```python
from build123d import *

# Parameters (mm, degrees)
SKETCH_1_W             = 140
SKETCH_1_H             = 60
EXTRUDE_1_DEPTH        = 5
SKETCH_2_R             = 1.2
CUT_EXTRUDE_1096_DEPTH = 153.397506541
SKETCH_4_R             = 1.4
CUT_EXTRUDE_3_DEPTH    = 5
PATTERN_LINEAR_1_COUNT = 3
PATTERN_LINEAR_1_PITCH = 40
SKETCH_6_R             = 2
CUT_EXTRUDE_4_DEPTH    = 1


with BuildPart() as part:
    # Sketch 1 → Extrude 1 (new body)
    with BuildSketch(Plane(origin=(0, 0, 0), x_dir=(1, 0, 0), z_dir=(0, 1, 0))):
        with Locations((70, -30)):
            Rectangle(SKETCH_1_W, SKETCH_1_H)
    extrude(amount=EXTRUDE_1_DEPTH)

    # Sketch 2 → Cut-Extrude 1096 (cut, through all)
    with BuildSketch(Plane(origin=(0, 5, 0), x_dir=(1, 0, 0), z_dir=(0, 1, 0))):
        with Locations(Location((102, -15, 0), (0, 0, 270))):
            Circle(SKETCH_2_R)
        with Locations(Location((118, -15, 0), (0, 0, 270))):
            Circle(SKETCH_2_R)
        with Locations(Location((102, -45, 0), (0, 0, 90))):
            Circle(SKETCH_2_R)
        with Locations(Location((118, -45, 0), (0, 0, 90))):
            Circle(SKETCH_2_R)
        with BuildLine():
            Line((100, -26.05), (100, -36.95))
            Line((100, -36.95), (104.2, -36.95))
            Line((104.2, -36.95), (104.2, -29.381860214))
            ThreePointArc((104.2, -29.381860214), (110, -31.5), (115.8, -29.381860214))
            Line((115.8, -29.381860214), (115.8, -36.95))
            Line((115.8, -36.95), (120, -36.95))
            Line((120, -36.95), (120, -26.05))
            Line((120, -26.05), (118.270278109, -26.05))
            ThreePointArc((118.270278109, -26.05), (110, -13.5), (101.729721891, -26.05))
            Line((101.729721891, -26.05), (100, -26.05))
        make_face()
    cut_extrude_1096 = extrude(amount=-CUT_EXTRUDE_1096_DEPTH, mode=Mode.SUBTRACT)

    # Sketch 4 → Cut-Extrude 3 (cut)
    with BuildSketch(Plane.ZY):
        with Locations((30, 2.5)):
            Circle(SKETCH_4_R)
        with Locations((8, 2.5)):
            Circle(SKETCH_4_R)
        with Locations((52, 2.5)):
            Circle(SKETCH_4_R)
    cut_extrude_3 = extrude(amount=-CUT_EXTRUDE_3_DEPTH, mode=Mode.SUBTRACT)

    # Mirror 1: Cut-Extrude 3 across plane
    add(cut_extrude_3.mirror(Plane(origin=(70, 0, 0), x_dir=(0, 0, 1), z_dir=(1, 0, 0))), mode=Mode.SUBTRACT)

    # Pattern Linear 1: Cut-Extrude 1096 ×3
    with Locations(*[(-i * PATTERN_LINEAR_1_PITCH, 0, 0) for i in range(1, PATTERN_LINEAR_1_COUNT)]):
        add(cut_extrude_1096, mode=Mode.SUBTRACT)

    # Sketch 6 → Cut-Extrude 4 (cut)
    with BuildSketch(Plane.XZ):
        with Locations(Location((22, 45, 0), (0, 0, 270))):
            Circle(SKETCH_6_R)
        with Locations(Location((38, 45, 0), (0, 0, 270))):
            Circle(SKETCH_6_R)
        with Locations(Location((62, 45, 0), (0, 0, 270))):
            Circle(SKETCH_6_R)
        with Locations(Location((78, 45, 0), (0, 0, 270))):
            Circle(SKETCH_6_R)
        with Locations(Location((102, 45, 0), (0, 0, 270))):
            Circle(SKETCH_6_R)
        with Locations(Location((118, 45, 0), (0, 0, 270))):
            Circle(SKETCH_6_R)
        with Locations((22, 15)):
            Circle(SKETCH_6_R)
        with Locations((38, 15)):
            Circle(SKETCH_6_R)
        with Locations((62, 15)):
            Circle(SKETCH_6_R)
        with Locations((78, 15)):
            Circle(SKETCH_6_R)
        with Locations((102, 15)):
            Circle(SKETCH_6_R)
        with Locations((118, 15)):
            Circle(SKETCH_6_R)
    extrude(amount=-CUT_EXTRUDE_4_DEPTH, mode=Mode.SUBTRACT)


solid = part.part
```
Could you check a few things on this model? Use its own coordinates, in mm. A direction names the side the tool comes from. Round coordinates to 2 decimals unless told otherwise and drop trailing zeros. Loops run counter-clockwise (first coordinate to the right, second up) from the corner with the lowest first, then second, coordinate; pieces in that order, holes last.
Q1. I want a section at B-B (y = 2.5). Give the number of separate pieces and of enclosed holes in the cut face, and give its area (3 significant figures).
Q2. On a 3-axis mill with a long thin cutter (end or side, diameter ignored), from which of +Z, -Z, +X, -X, +Y, -Y can I reach the whole of each face in a straight line? I mean faces 1 (the flat face through (23, 1, 14)), 2 (the flat face through (104.2, 3, 33)), 3 (the cylindrical face through (137.54, 1.96, 53.29)). Say none if no direction works.
Q3. Please list where these lines run through material, in increasing order: L1, parallel to Z at x = 30, y = 1.8; L2, parallel to Y at x = 137, z = 52; L3, parallel to Z at x = 118, y = 3.2.
Q4. Thinking about a two-plate mould opening in X: for faces 4 (the flat face through (69, 5, 36)), 5 (the flat face through (135, 3, 30)), 6 (the cylindrical face through (60.99, 3.03, 44.35)), which applies, pulls with the +X half, pulls with the -X half, needs draft (parallel to the pull), parting line crosses it, or undercut?
Q5. For P1, Ø3, axis at x = 22, z = 15, coming from the -Y side; P2, Ø2, axis at x = 102, z = 45, coming from the -Y side, each with a flat end and sliding along its axis, tell me the tip position at first contact or that it passes through.
Q6. I want a section at A-A (z = 8). Write out the boundary of the cut face in (x, y), and give its area (3 significant figures).
Answer below:
1. separate pieces: 1
1. enclosed holes: 15
1. area: 7,250 mm2
2. face 1: -Y
2. face 2: +Y, -Y
2. face 3: +X
3. L1: z = 0 to 13.5, 31.5 to 60
3. L2: y = 0 to 1.1, 3.9 to 5
3. L3: z = 0 to 13.8, 16.2 to 18.38, 36.95 to 43.8, 46.2 to 60
4. face 4: needs draft
4. face 5: pulls with the +X half
4. face 6: undercut
5. P1: stops at y = 1
5. P2: passes through
6. outline: (0, 0) - (140, 0) - (140, 1.1) - (135, 1.1) - (135, 3.9) - (140, 3.9) - (140, 5) - (0, 5) - (0, 3.9) - (5, 3.9) - (5, 1.1) - (0, 1.1) - close
6. area: 672 mm2
